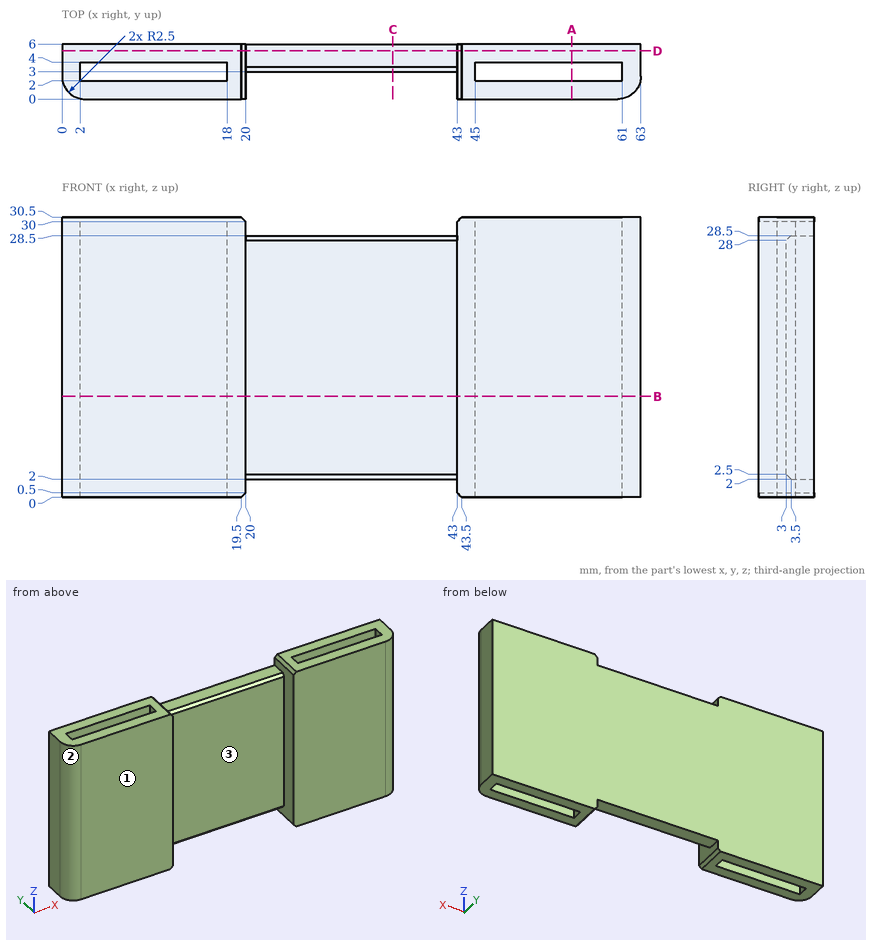
Drawing for the job (mm, zero at the part's lowest x, y, z). Round coordinates to 2 decimals unless told otherwise and drop trailing zeros. Write each loop counter-clockwise with the first axis right and the second up, starting at its lowest first coordinate (ties: lowest second). Pieces come first, ordered by that corner, then holes. Notation, with made-up numbers: M -18,-9.75 L -8,-9.75 A19 cw -8,-1.75 Z; hole C -20.75,17 d6. An arc over 180 degrees is marked long. Put each result on its own line as item: value.
Item 1: Cut at B-B (z = 11). List the corners of the cut face in (x, y).
Responses:
outline: M 0,2.5 A2.5 ccw 2.5,0 L 20,0 L 20,3 L 43,3 L 43,0 L 60.5,0 A2.5 ccw 63,2.5 L 63,6 L 0,6 Z; hole M 2,2 L 18,2 L 18,4 L 2,4 Z; hole M 45,2 L 61,2 L 61,4 L 45,4 Z
Item 2: Flat gauge pins, fed straight in: P1, Ø1.5, axis at x = 26, y = 5.5, coming from the -Z side; P2, Ø2, axis at y = 2.5, z = 13, coming from the -X side; P3, Ø7, axis at x = 29, z = 19, coming from the -Y side; P4, Ø2, axis at x = 35, y = 4, coming from the +Z side. Where does each tip first touch, or does it go through?
Responses:
P1: z = 2
P2: x = 0
P3: y = 3
P4: z = 28.5
Item 3: Cut at D-D (y = 5.25). List the corners of the cut face in (x, z), and give its area (3 significant figures).
Responses:
outline: M 0,0 L 19.5,0 L 20,0.5 L 20,2 L 43,2 L 43,0.5 L 43.5,0 L 63,0 L 63,30.5 L 43.5,30.5 L 43,30 L 43,28.5 L 20,28.5 L 20,30 L 19.5,30.5 L 0,30.5 Z
area: 1,830 mm²
Item 4: Cut at A-A (x = 55.5). List the corners of the cut face in (y, z).
Responses:
outline: M 0,0 L 2,0 L 2,30.5 L 0,30.5 Z; M 4,0 L 6,0 L 6,30.5 L 4,30.5 Z
Item 5: Cut at C-C (x = 36). List the corners of the cut face in (y, z), and give its area (4 significant figures).
Responses:
outline: M 3,2.5 L 3.5,2 L 6,2 L 6,28.5 L 3.5,28.5 L 3,28 Z
area: 79.25 mm²
Item 6: Probe L1, parallel to X at y = 3, z = 29.5; L2, parallel to Y at x = 7.5, z = 23; L3, parallel to Y at x = 37, z = 20.5. List the from-to ranges inside material, lowest first. Write a range as from..to.
Responses:
L1: 0..2, 18..20, 43..45, 61..63
L2: 0..2, 4..6
L3: 3..6
Item 7: Mould opens along X. For the marked faces 1, 2 and 3 say: +X half, -X half, draft (parallel to the pull), parting line (faces both ways), or undercut.
Responses:
face 1: draft
face 2: -X half
face 3: undercut
